```python
from build123d import *

# Parameters (mm, degrees)
F1_DEPTH = 32
F3_DEPTH = 1.2
F7_DEPTH = 5
F8_DEPTH = 5


with BuildPart() as f1:
    # F0 (on Top) → F1 (new body)
    with BuildSketch(Plane.XY):
        Polygon((-18.723475383, -22.2), (-11.323475383, -22.2), (-11.323475383, -14.2), (-2.25, -14.2), (2.25, -14.2), (11.323475383, -14.2), (11.323475383, -22.2), (18.723475383, -22.2), (18.723475383, 0), (18.723475383, 22.2), (11.323475383, 22.2), (11.323475383, 10.2626532034), (-4.423475383, 10.2626532034), (-6.823475383, 10.2626532034), (-11.323475383, 10.2626532034), (-11.323475383, 22.2), (-18.723475383, 22.2), (-18.723475383, 0), align=None)
        with BuildLine():
            ThreePointArc((-2.25, -6.0981554588), (-3.833092601, -5.2495143691), (-5.123475383, -4))
            Line((-5.123475383, -4), (-8.523475383, -2.9))
            Line((-8.523475383, -2.9), (-10.323475383, -2.9))
            Line((-10.323475383, -2.9), (-10.323475383, -4))
            Line((-10.323475383, -4), (-10.723475383, -4))
            Line((-10.723475383, -4), (-10.723475383, -7))
            Line((-10.723475383, -7), (-12.523475383, -7))
            Line((-12.523475383, -7), (-12.523475383, -21))
            Line((-12.523475383, -21), (-17.523475383, -21))
            Line((-17.523475383, -21), (-17.523475383, 0))
            Line((-17.523475383, 0), (-17.523475383, 21))
            Line((-17.523475383, 21), (-12.523475383, 21))
            Line((-12.523475383, 21), (-12.523475383, 7))
            Line((-12.523475383, 7), (-10.723475383, 7))
            Line((-10.723475383, 7), (-10.723475383, 4))
            Line((-10.723475383, 4), (-10.323475383, 4))
            Line((-10.323475383, 4), (-10.323475383, 2.9))
            Line((-10.323475383, 2.9), (-8.523475383, 2.9))
            Line((-8.523475383, 2.9), (-6.823475383, 3.45))
            Line((-6.823475383, 3.45), (-6.823475383, 9.0626532034))
            Line((-6.823475383, 9.0626532034), (-4.423475383, 9.0626532034))
            Line((-4.423475383, 9.0626532034), (-4.423475383, 4.7626532034))
            ThreePointArc((-4.423475383, 4.7626532034), (-2.5613294597, 5.9740766148), (-0.4, 6.4876806333))
            Line((-0.4, 6.4876806333), (-0.4, 7.3))
            Line((-0.4, 7.3), (0, 7.3))
            Line((0, 7.3), (0.4, 7.3))
            Line((0.4, 7.3), (0.4, 6.4876806333))
            ThreePointArc((0.4, 6.4876806333), (3.0289162765, 5.7511447721), (5.123475383, 4))
            Line((5.123475383, 4), (8.523475383, 2.9))
            Line((8.523475383, 2.9), (10.323475383, 2.9))
            Line((10.323475383, 2.9), (10.323475383, 4))
            Line((10.323475383, 4), (10.723475383, 4))
            Line((10.723475383, 4), (10.723475383, 7))
            Line((10.723475383, 7), (12.523475383, 7))
            Line((12.523475383, 7), (12.523475383, 21))
            Line((12.523475383, 21), (17.523475383, 21))
            Line((17.523475383, 21), (17.523475383, 0))
            Line((17.523475383, 0), (17.523475383, -21))
            Line((17.523475383, -21), (12.523475383, -21))
            Line((12.523475383, -21), (12.523475383, -7))
            Line((12.523475383, -7), (10.723475383, -7))
            Line((10.723475383, -7), (10.723475383, -4))
            Line((10.723475383, -4), (10.323475383, -4))
            Line((10.323475383, -4), (10.323475383, -2.9))
            Line((10.323475383, -2.9), (8.523475383, -2.9))
            Line((8.523475383, -2.9), (5.123475383, -4))
            ThreePointArc((5.123475383, -4), (3.833092601, -5.2495143691), (2.25, -6.0981554588))
            Line((2.25, -6.0981554588), (2.25, -13))
            Line((2.25, -13), (-2.25, -13))
            Line((-2.25, -13), (-2.25, -6.0981554588))
        make_face(mode=Mode.SUBTRACT)
    extrude(amount=F1_DEPTH)

    # F2 (on face) → F3 (join)
    with BuildSketch(Plane(origin=(0, 0, 0), x_dir=(1, 0, 0), z_dir=(0, 0, -1))):
        Polygon((11.323475383, -10.2626532034), (11.323475383, -22.2), (18.723475383, -22.2), (18.723475383, 0), (18.723475383, 22.2), (11.323475383, 22.2), (11.323475383, 14.2), (-11.323475383, 14.2), (-11.323475383, 22.2), (-18.723475383, 22.2), (-18.723475383, -22.2), (-11.323475383, -22.2), (-11.323475383, -10.2626532034), align=None)
        with BuildLine():
            Line((17.523475383, 21), (17.523475383, 0))
            Line((17.523475383, 0), (17.523475383, -21))
            Line((17.523475383, -21), (12.523475383, -21))
            Line((12.523475383, -21), (12.523475383, -7))
            Line((12.523475383, -7), (10.723475383, -7))
            Line((10.723475383, -7), (10.723475383, -4))
            Line((10.723475383, -4), (10.323475383, -4))
            Line((10.323475383, -4), (10.323475383, -2.9))
            Line((10.323475383, -2.9), (8.523475383, -2.9))
            Line((8.523475383, -2.9), (5.123475383, -4))
            ThreePointArc((5.123475383, -4), (3.0289162765, -5.7511447721), (0.4, -6.4876806333))
            Line((0.4, -6.4876806333), (0.4, -7.3))
            Line((0.4, -7.3), (-0.4, -7.3))
            Line((-0.4, -7.3), (-0.4, -6.4876806333))
            ThreePointArc((-0.4, -6.4876806333), (-2.5613294597, -5.9740766148), (-4.423475383, -4.7626532034))
            Line((-4.423475383, -4.7626532034), (-4.423475383, -9.0626532034))
            Line((-4.423475383, -9.0626532034), (-6.823475383, -9.0626532034))
            Line((-6.823475383, -9.0626532034), (-6.823475383, -3.45))
            Line((-6.823475383, -3.45), (-8.523475383, -2.9))
            Line((-8.523475383, -2.9), (-10.323475383, -2.9))
            Line((-10.323475383, -2.9), (-10.323475383, -4))
            Line((-10.323475383, -4), (-10.723475383, -4))
            Line((-10.723475383, -4), (-10.723475383, -7))
            Line((-10.723475383, -7), (-12.523475383, -7))
            Line((-12.523475383, -7), (-12.523475383, -21))
            Line((-12.523475383, -21), (-17.523475383, -21))
            Line((-17.523475383, -21), (-17.523475383, 0))
            Line((-17.523475383, 0), (-17.523475383, 21))
            Line((-17.523475383, 21), (-12.523475383, 21))
            Line((-12.523475383, 21), (-12.523475383, 7))
            Line((-12.523475383, 7), (-10.723475383, 7))
            Line((-10.723475383, 7), (-10.723475383, 4))
            Line((-10.723475383, 4), (-10.323475383, 4))
            Line((-10.323475383, 4), (-10.323475383, 2.9))
            Line((-10.323475383, 2.9), (-8.523475383, 2.9))
            Line((-8.523475383, 2.9), (-5.123475383, 4))
            ThreePointArc((-5.123475383, 4), (-3.833092601, 5.2495143691), (-2.25, 6.0981554588))
            Line((-2.25, 6.0981554588), (-2.25, 13))
            Line((-2.25, 13), (2.25, 13))
            Line((2.25, 13), (2.25, 6.0981554588))
            ThreePointArc((2.25, 6.0981554588), (3.833092601, 5.2495143691), (5.123475383, 4))
            Line((5.123475383, 4), (8.523475383, 2.9))
            Line((8.523475383, 2.9), (10.323475383, 2.9))
            Line((10.323475383, 2.9), (10.323475383, 4))
            Line((10.323475383, 4), (10.723475383, 4))
            Line((10.723475383, 4), (10.723475383, 7))
            Line((10.723475383, 7), (12.523475383, 7))
            Line((12.523475383, 7), (12.523475383, 21))
            Line((12.523475383, 21), (17.523475383, 21))
        make_face(mode=Mode.SUBTRACT)
        with BuildLine():
            Line((17.523475383, -21), (17.523475383, 0))
            Line((17.523475383, 0), (-17.523475383, 0))
            Line((-17.523475383, 0), (-17.523475383, -21))
            Line((-17.523475383, -21), (-12.523475383, -21))
            Line((-12.523475383, -21), (-12.523475383, -7))
            Line((-12.523475383, -7), (-10.723475383, -7))
            Line((-10.723475383, -7), (-10.723475383, -4))
            Line((-10.723475383, -4), (-10.323475383, -4))
            Line((-10.323475383, -4), (-10.323475383, -2.9))
            Line((-10.323475383, -2.9), (-8.523475383, -2.9))
            Line((-8.523475383, -2.9), (-6.823475383, -3.45))
            Line((-6.823475383, -3.45), (-6.823475383, -9.0626532034))
            Line((-6.823475383, -9.0626532034), (-4.423475383, -9.0626532034))
            Line((-4.423475383, -9.0626532034), (-4.423475383, -4.7626532034))
            ThreePointArc((-4.423475383, -4.7626532034), (-2.5613294597, -5.9740766148), (-0.4, -6.4876806333))
            Line((-0.4, -6.4876806333), (-0.4, -7.3))
            Line((-0.4, -7.3), (0.4, -7.3))
            Line((0.4, -7.3), (0.4, -6.4876806333))
            ThreePointArc((0.4, -6.4876806333), (3.0289162765, -5.7511447721), (5.123475383, -4))
            Line((5.123475383, -4), (8.523475383, -2.9))
            Line((8.523475383, -2.9), (10.323475383, -2.9))
            Line((10.323475383, -2.9), (10.323475383, -4))
            Line((10.323475383, -4), (10.723475383, -4))
            Line((10.723475383, -4), (10.723475383, -7))
            Line((10.723475383, -7), (12.523475383, -7))
            Line((12.523475383, -7), (12.523475383, -21))
            Line((12.523475383, -21), (17.523475383, -21))
        make_face()
        with BuildLine():
            Line((-17.523475383, 0), (17.523475383, 0))
            Line((17.523475383, 0), (17.523475383, 21))
            Line((17.523475383, 21), (12.523475383, 21))
            Line((12.523475383, 21), (12.523475383, 7))
            Line((12.523475383, 7), (10.723475383, 7))
            Line((10.723475383, 7), (10.723475383, 4))
            Line((10.723475383, 4), (10.323475383, 4))
            Line((10.323475383, 4), (10.323475383, 2.9))
            Line((10.323475383, 2.9), (8.523475383, 2.9))
            Line((8.523475383, 2.9), (5.123475383, 4))
            ThreePointArc((5.123475383, 4), (3.833092601, 5.2495143691), (2.25, 6.0981554588))
            Line((2.25, 6.0981554588), (2.25, 13))
            Line((2.25, 13), (-2.25, 13))
            Line((-2.25, 13), (-2.25, 6.0981554588))
            ThreePointArc((-2.25, 6.0981554588), (-3.833092601, 5.2495143691), (-5.123475383, 4))
            Line((-5.123475383, 4), (-8.523475383, 2.9))
            Line((-8.523475383, 2.9), (-10.323475383, 2.9))
            Line((-10.323475383, 2.9), (-10.323475383, 4))
            Line((-10.323475383, 4), (-10.723475383, 4))
            Line((-10.723475383, 4), (-10.723475383, 7))
            Line((-10.723475383, 7), (-12.523475383, 7))
            Line((-12.523475383, 7), (-12.523475383, 21))
            Line((-12.523475383, 21), (-17.523475383, 21))
            Line((-17.523475383, 21), (-17.523475383, 0))
        make_face()
    extrude(amount=F3_DEPTH)

    # F5 (on face) → F7 (join, through all)
    with BuildSketch(Plane.YZ.offset(-17.523475383)):
        Polygon((-21, 4), (-21, 0), (0, 0), align=None)
        Polygon((21, 4), (0, 0), (21, 0), align=None)
    extrude(amount=F7_DEPTH)

    # F6 (on face) → F8 (join, through all)
    with BuildSketch(Plane(origin=(17.523475383, 0, 0), x_dir=(0, -1, 0), z_dir=(-1, 0, 0))):
        Polygon((-21, 4), (-21, 0), (0, 0), align=None)
        Polygon((21, 4), (0, 0), (21, 0), align=None)
    extrude(amount=F8_DEPTH)


solid = f1.part
```
Design review of the part built by this model. Coordinates are the model's own, in mm. A direction names the side the tool comes from. Coordinates: 2 decimals unless noted, no trailing zeros. Loops run counter-clockwise (first coordinate to the right, second up) from the corner with the lowest first, then second, coordinate; pieces in that order, holes last.
Q1. We need section A-A on x = -16. State the section outline as (y, z) points, and give its area (3 significant figures).
Reported:
outline: (-22.2, -1.2) - (22.2, -1.2) - (22.2, 32) - (21, 32) - (21, 4) - (0, 0) - (-21, 4) - (-21, 32) - (-22.2, 32) - close
area: 214 mm2
Q2. The part is to be moulded in two halves that separate along X. For faces 1 (the face through (15, -22.2, 16)), 2 (the face through (10.323, -3.5, 15.8)), 3 (the face through (-18.723, 0, 16)), say which applies: +X half, -X half, draft (parallel to the pull), parting line (faces both ways), or undercut.
Reported:
face 1: draft
face 2: undercut
face 3: -X half
Q3. We need section C-C on x = -9.5. State the section outline as (y, z) points, and give its area (3 significant figures).
Reported:
outline: (-14.2, -1.2) - (10.26, -1.2) - (10.26, 32) - (2.9, 32) - (2.9, 0) - (-2.9, 0) - (-2.9, 32) - (-14.2, 32) - close
area: 627 mm2
Q4. To check wall thickness, follow line 1 (X direction, y = -15.5, z = 22.5); line 2 (X direction, y = -8, z = 26); line 3 (Y direction, x = -16, z = 29). State the ranges of each line that lie inside material, in increasing order.
Reported:
line 1: x = -18.72 to -17.52, -12.52 to -11.32, 11.32 to 12.52, 17.52 to 18.72
line 2: x = -18.72 to -17.52, -12.52 to -2.25, 2.25 to 12.52, 17.52 to 18.72
line 3: y = -22.2 to -21, 21 to 22.2
Q5. We need section B-B on y = 11. State the section outline as (x, z) points.
Reported:
outline: (-18.72, -1.2) - (-11.32, -1.2) - (-11.32, 32) - (-12.52, 32) - (-12.52, 2.1) - (-17.52, 2.1) - (-17.52, 32) - (-18.72, 32) - close; (11.32, -1.2) - (18.72, -1.2) - (18.72, 32) - (17.52, 32) - (17.52, 2.1) - (12.52, 2.1) - (12.52, 32) - (11.32, 32) - close
Q6. For pin 1 (0.5 mm diameter, centred on x = -9, z = 21, fed in from -Y); pin 2 (4 mm diameter, centred on x = -4.5, y = -15.5, fed in from +Z), all flat-tipped, find the tip position at first contact; note any pin that passes through.
Reported:
pin 1: stops at y = -14.2
pin 2: stops at z = 32
Q7. We need section D-D on x = 1. State the section outline as (y, z) points, and give its area (3 significant figures).
Reported:
outline: (-14.2, -1.2) - (10.26, -1.2) - (10.26, 32) - (6.42, 32) - (6.42, 0) - (-13, 0) - (-13, 32) - (-14.2, 32) - close
area: 191 mm2
Q8. Tool access review of faces 4 (the face through (-15, 22.2, 16)), 5 (the face through (-6.823, 6, 16)): name each direction out of +Z, -Z, +X, -X, +Y, -Y from which nothing blocks a thin tool from reaching the whole face with its end or side.
Reported:
face 4: +Z, -Z, +X, -X, +Y
face 5: +Z
